Work out the finished part from the listing and answer in its coordinate system (mm). A direction names the side the tool comes from. Give positions to 0.01 mm unless a question says otherwise; leave off trailing zeros. Loops run counter-clockwise (first coordinate to the right, second up) from the corner with the lowest first, then second, coordinate; pieces in that order, holes last. Notation, with made-up numbers: M 80.5,4.25 L 126.5,4.25 A3 cw 126.5,8.25 Z; hole C 71.5,25 d2. An arc over 180 degrees is marked long. Write item = value, one per line. Start each with the question number.
1. Consider L1, parallel to X at y = -174.6, z = 3.65; L2, parallel to X at y = -174.6, z = 4.9; L3, parallel to Y at x = 99.16, z = 4.2. Determine where each line is inside the solid, lowest interval first. Write a range as [from, to].
2. Flat-ended cylindrical pins translate along their axes: pin 1 Ø2.5 at (x, y) = (99, -185.5) entering from +Z; pin 2 Ø3 at (x, z) = (105, 5) entering from +Y; pin 3 Ø2.5 at (x, y) = (98.5, -163.5) entering from +Z. Find the tip coordinate at first contact, or state that the pin passes through.
3. The mould has two halves that part along X. Classify faces 1 (the face through (99.1, -186.7, 3)), 2 (the face through (103, -172, 10.5)), 3 (the face through (103.49, -174.79, 10.25)): released by +X, released by -X, zero draft, split by the parting line, or undercut.
4. Section C-C on y = -174.6 is taken. Determine the outline of the cut face in (x, z).
5. Section B-B on x = 99.16 is taken. Determine the outline of the cut face in (y, z), plus the area to 3 significant figures.
6. For faces 4 (the face through (99.84, -179.81, 10.32)), 5 (the face through (100.38, -183.92, 3.96)), determine the directions among +Z, -Z, +X, -X, +Y, -Y from which every point of the face is accessible in a straight line to the end or side of a thin tool.
7. Section A-A on z = 3.75 is taken. Determine the outline of the cut face in (x, y).
8. Section D-D on z = 5.5 is taken. Determine the outline of the cut face in (x, y).
```python
from build123d import *

# Parameters (mm, degrees)
PAD022_DEPTH          = 3
POLARPATTERN001_COUNT = 4


with BuildPart() as part:
    # Sketch042 → Revolution002 (revolve)
    with BuildSketch(Plane.XZ):
        Polygon((-10, 0), (-10, 5.302235), (-5.008018, 9), (-4, 9), (-9.4, 5), (-9.4, 0), align=None)
    revolve(axis=Axis((0, 0, 0), (0, 0, 1)))

    # Sketch043 → Pad022 (new body)
    with BuildSketch(Plane.XY):
        with BuildLine():
            ThreePointArc((-10.3, 1.8), (-12.1, 0), (-10.3, -1.8))
            Line((-10.3, -1.8), (-9.6, -1.8))
            Line((-9.6, -1.8), (-9.6, 1.8))
            Line((-9.6, 1.8), (-10.3, 1.8))
        make_face()
        with BuildLine():
            ThreePointArc((10.3, -1.8), (12.1, 0), (10.3, 1.8))
            Line((10.3, 1.8), (9.6, 1.8))
            Line((9.6, 1.8), (9.6, -1.8))
            Line((10.3, -1.8), (9.6, -1.8))
        make_face()
    pad022 = extrude(amount=PAD022_DEPTH)

    # PolarPattern001: Pad022 ×4 about axis
    polarpattern001_axis = Axis((0, 0, 0), (0, 0, 1))
    for i in range(1, POLARPATTERN001_COUNT):
        add(pad022.rotate(polarpattern001_axis, i * 360 / POLARPATTERN001_COUNT))


with BuildPart() as part_1:
    # Body007 placement: moved
    add(part.part.moved(Location((99.16, -174.6, 1.5))))


solid = part_1.part
```
Verdict:
q1.L1 = [87.06, 89.76], [108.56, 111.26]
q1.L2 = [89.16, 89.76], [108.56, 109.16]
q1.L3 = [-186.7, -184], [-165.2, -162.5]
q2.pin_1 = 7.06
q2.pin_2 = -165.59
q2.pin_3 = 6.9
q3.face_1 = split by the parting line
q3.face_2 = zero draft
q3.face_3 = undercut
q4.outline = M 87.06,1.5 L 89.76,1.5 L 89.76,6.5 L 95.16,10.5 L 94.15,10.5 L 89.16,6.8 L 89.16,4.5 L 87.06,4.5 Z; M 103.16,10.5 L 108.56,6.5 L 108.56,1.5 L 111.26,1.5 L 111.26,4.5 L 109.16,4.5 L 109.16,6.8 L 104.17,10.5 Z
q5.outline = M -186.7,1.5 L -184,1.5 L -184,6.5 L -178.6,10.5 L -179.61,10.5 L -184.6,6.8 L -184.6,4.5 L -186.7,4.5 Z; M -170.6,10.5 L -165.2,6.5 L -165.2,1.5 L -162.5,1.5 L -162.5,4.5 L -164.6,4.5 L -164.6,6.8 L -169.59,10.5 Z
q5.area = 26.5 mm2
q6.face_4 = +Z
q6.face_5 = -Z
q7.outline = M 88.86,-176.4 L 89.32,-176.4 A10 ccw 97.36,-184.44 L 97.36,-184.9 A1.8 ccw 100.96,-184.9 L 100.96,-184.44 A10 ccw 109,-176.4 L 109.46,-176.4 A1.8 ccw 109.46,-172.8 L 109,-172.8 A10 ccw 100.96,-164.76 L 100.96,-164.3 A1.8 ccw 97.36,-164.3 L 97.36,-164.76 A10 ccw 89.32,-172.8 L 88.86,-172.8 A1.8 ccw Z; hole C 99.16,-174.6 d18.8
q8.outline = C 99.16,-174.6 d20; hole C 99.16,-174.6 d18.8
